Build history of the part. All positions in model axes, mm. Face numbers are marked on the shaded views. A direction names the side the tool comes from. Give positions to 0.01 mm unless a question says otherwise; leave off trailing zeros. Write each loop counter-clockwise with the first axis right and the second up, starting at its lowest first coordinate (ties: lowest second). Pieces come first, ordered by that corner, then holes. Notation, with made-up numbers: (54, 19) -> (71, 19) arc R17 cw to (71, 52) -> close; hole circle Ø4 at (-22, -8). An arc over 180 degrees is marked (long way). One line per question, with ' | ' between items. Start each with the question number.
(1) Band-saw the part on A-A, the plane y = -1.25. Give the cut face in (x, z) (3 decimals).
(2) Drill centre lines: probe 1 along X at (y, z) = (-1.95, 0); probe 2 along X at (y, z) = (-3.1, 0) (3 decimals); probe 3 along Z at (x, y) = (-0.25, -2.9). Where is each one in solid material? Low to high. Write a range as from..to.
(3) Pull direction X, two halves, no side cores. Call the marked faces 4, 5 and 6: released by +X, released by -X, zero draft, split by the parting line, or undercut.
(4) Pin check, flat tips, straight feed: P1, Ø2, axis at x = 0, y = -1.5, coming from the +Z side (3 decimals); P2, Ø1.5, axis at x = -2.5, y = -1, coming from the -Z side; P3, Ø3, axis at x = 0.5, z = 0, coming from the +Y side. Stop position of each tip, or through.
(5) Tool access for the marked faces 1, 2 and 3: list every direction of +Z, -Z, +X, -X, +Y, -Y with a clear straight run to the whole face (end or side of a thin tool).
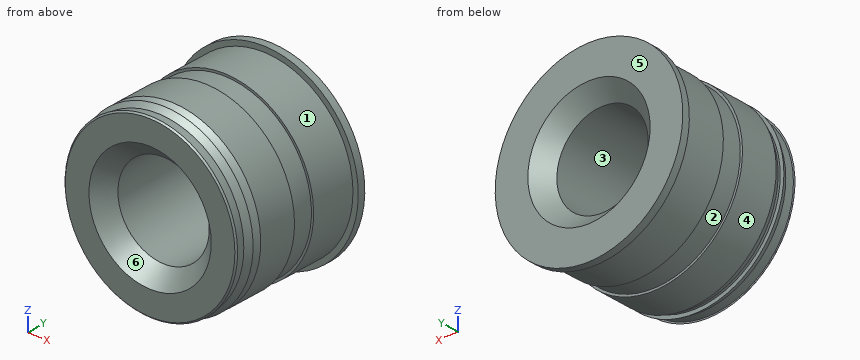
from build123d import *

# Parameters (mm, degrees)
SKETCH1_R      = 2.87
EXTRUDE1_DEPTH = 4.7
SKETCH1_4_R    = 2.995
EXTRUDE2_DEPTH = 3.838846
SKETCH1_3_R    = 3.175
EXTRUDE3_DEPTH = 0.254
SKETCH2_R      = 2.995
EXTRUDE4_DEPTH = 0.216506
EXTRUDE4_TAPER = 30
SKETCH8_R      = 1.545336663
EXTRUDE6_DEPTH = 4.7
CHAMFER1_SIZE  = 0.525
SKETCH11_W     = 0.255
SKETCH11_H     = 0.74295


# Read off the part's stored shape, not the designer's step: Extrude5
with BuildPart() as part:
    # Sketch1 → Extrude1 (new body)
    with BuildSketch(Plane(origin=(0, 0, 0), x_dir=(1, 0, 0), z_dir=(0, 1, 0))):
        with Locations(Location((0, 0, 0), (0, 0, 270))):
            Circle(SKETCH1_R)
    extrude(amount=-EXTRUDE1_DEPTH)

    # Sketch1<4> → Extrude2 (add)
    with BuildSketch(Plane(origin=(0, 0, 0), x_dir=(1, 0, 0), z_dir=(0, 1, 0))):
        with Locations(Location((0, 0, 0), (0, 0, 270))):
            Circle(SKETCH1_4_R)
    extrude(amount=-EXTRUDE2_DEPTH)

    # Sketch1<3> → Extrude3 (add)
    with BuildSketch(Plane(origin=(0, 0, 0), x_dir=(1, 0, 0), z_dir=(0, 1, 0))):
        with Locations(Location((0, 0, 0), (0, 0, 270))):
            Circle(SKETCH1_3_R)
    extrude(amount=-EXTRUDE3_DEPTH)

    # Sketch2 → Extrude4 (add)
    with BuildSketch(Plane.XZ.offset(3.838846189)):
        with Locations(Location((0, 0, 0), (0, 0, 90))):
            Circle(SKETCH2_R)
    extrude(amount=EXTRUDE4_DEPTH, taper=EXTRUDE4_TAPER)

    # Extrude5 outline → Extrude5 (revolve)
    with BuildSketch(Plane.XY):
        Polygon((2.87, -4.65), (2.87, -4.7), (2.92, -4.65), align=None)
    revolve(axis=Axis((0, 0, 0), (0, 1, 0)))

    # Sketch5 → Revolve1 (revolve)
    with BuildSketch(Plane.XY):
        Polygon((-2.87, -4.35267627), (-2.995, -4.136169919), (-2.87, -4.136169919), align=None)
    revolve(axis=Axis((0, 0, 0), (0, -1, 0)))

    # Sketch8 → Extrude6 (cut)
    with BuildSketch(Plane(origin=(0, 0, 0), x_dir=(1, 0, 0), z_dir=(0, 1, 0))):
        with Locations(Location((0, 0, 0), (0, 0, 270))):
            Circle(SKETCH8_R)
    extrude(amount=-EXTRUDE6_DEPTH, mode=Mode.SUBTRACT)

    # Chamfer1
    chamfer1_edges = [part.edges().sort_by_distance(p)[0] for p in [
        (0, -4.7, -1.545336663),
        (0, 0, -1.545336663),
    ]]
    chamfer(chamfer1_edges, length=CHAMFER1_SIZE)

    # Sketch11 → Cut-Revolve1 (revolve, cut)
    with BuildSketch(Plane.XY):
        with Locations((-3.0475, -2.15467627)):
            Rectangle(SKETCH11_W, SKETCH11_H)
    revolve(axis=Axis((0, 0, 0), (0, -1, 0)), mode=Mode.SUBTRACT)


solid = part.part
Results:
1) outline: circle Ø5.99 at (0, 0); hole circle Ø3.091 at (0, 0)
2) probe 1: x = -2.92..-1.55, 1.55..2.92 | probe 2: x = -2.995..-1.545, 1.545..2.995 | probe 3: z = -2.98..-1.52, 1.52..2.98
3) face 4: split by the parting line | face 5: zero draft | face 6: undercut
4) P1: stops at z = 2.995 | P2: stops at z = -2.43 | P3: stops at y = -0.07
5) face 1: -Y | face 2: none | face 3: +Y, -Y
